```python
from build123d import *

# Parameters (mm, degrees)
F0_W     = 50.8
F0_H     = 50.8
F0_W_2   = 46.8
F0_H_2   = 46.8
F1_DEPTH = 3.175
F2_DEPTH = 200.025


with BuildPart() as f1:
    # F0 (on Top) → F1 (new body)
    with BuildSketch(Plane.XY):
        Rectangle(F0_W, F0_H)
        Rectangle(F0_W_2, F0_H_2, mode=Mode.SUBTRACT)
        Rectangle(F0_W_2, F0_H_2)
    extrude(amount=F1_DEPTH)

    # F0 (on Top) → F2 (join)
    with BuildSketch(Plane.XY):
        Rectangle(F0_W, F0_H)
        Rectangle(F0_W_2, F0_H_2, mode=Mode.SUBTRACT)
    extrude(amount=-F2_DEPTH)


solid = f1.part
```
The listing builds one solid part. Answer for the finished solid, in the listing's coordinates (mm). A direction names the side the tool comes from. Coordinates: 2 decimals unless noted, no trailing zeros. Loops run counter-clockwise (first coordinate to the right, second up) from the corner with the lowest first, then second, coordinate; pieces in that order, holes last. Notation, with made-up numbers: (63, 26.25) - (101, 26.25) arc R14 ccw to (101, 39.25) - close; hole circle Ø10 at (-28.5, 16.25). An arc over 180 degrees is marked (long way). Use a Markdown table: item, result. Add a question column.
1) Given pin 1 (23.5 mm diameter, centred on x = 8.5, y = 4, fed in from -Z), flat-ended and moving along its own axis, determine where the tip first touches the part or whether it passes through.
2) For faces 1 (the flat face through (23.4, 0, -99)), 2 (the flat face through (0, 0, 3.175)), determine the directions among +Z, -Z, +X, -X, +Y, -Y from which every point of the face is accessible in a straight line to the end or side of a thin tool.
3) The part is cut by section B-B, the plane y = -12. Give the vertices of the cut face in (x, z) (3 decimals).
4) The mould has two halves that part along Y. Classify faces 3 (the flat face through (-23.4, 0, -99)), 4 (the flat face through (0, 23.4, -99)), 5 (the flat face through (-25.4, 0, -97)), 6 (the flat face through (0, 25.4, -97)): released by +Y, released by -Y, zero draft, split by the parting line, or undercut.
5) Find the intervals of material crossed by line 1 (X direction, y = 17, z = -70.5); line 2 (Z direction, x = -19, y = 7.5) (3 decimals), in increasing order.
6) The part is cut by section A-A, the plane z = -119.5. Give the vertices of the cut face in (x, y), and give its area (3 significant figures).
Here are the results:
| question | item | result |
|---|---|---|
| 1 | pin 1 | stops at z = 0 |
| 2 | face 1 | -Z |
| 2 | face 2 | +Z, +X, -X, +Y, -Y |
| 3 | outline | (-25.4, -200.025) - (-23.4, -200.025) - (-23.4, 0) - (23.4, 0) - (23.4, -200.025) - (25.4, -200.025) - (25.4, 3.175) - (-25.4, 3.175) - close |
| 4 | face 3 | undercut |
| 4 | face 4 | undercut |
| 4 | face 5 | zero draft |
| 4 | face 6 | released by +Y |
| 5 | line 1 | x = -25.4 to -23.4, 23.4 to 25.4 |
| 5 | line 2 | z = 0 to 3.175 |
| 6 | outline | (-25.4, -25.4) - (25.4, -25.4) - (25.4, 25.4) - (-25.4, 25.4) - close; hole (-23.4, -23.4) - (23.4, -23.4) - (23.4, 23.4) - (-23.4, 23.4) - close |
| 6 | area | 390 mm^2 |
